```python
from build123d import *

# Parameters (mm, degrees)
SKETCH1_R               = 12.5
BOSS_EXTRUDE1_DEPTH     = 22.5
SKETCH2_R               = 7.5
CUT_EXTRUDE2_DEPTH      = 18.320508076
CUT_EXTRUDE2_DEPTH_BACK = 18.320508076
BOSS_EXTRUDE2_START     = -5
SKETCH3_R               = 12.5
BOSS_EXTRUDE2_DEPTH     = 15
SKETCH4_R               = 17.320508076
BOSS_EXTRUDE3_DEPTH     = 5


with BuildPart() as part:
    # Sketch1 → Boss-Extrude1 (new body, symmetric)
    with BuildSketch(Plane(origin=(0, 0, 0), x_dir=(0, 0, -1), z_dir=(1, 0, 0))):
        Polygon((10, 17.320508076), (-10, 17.320508076), (-20, 0), (-10, -17.320508076), (10, -17.320508076), (20, 0), align=None)
        Circle(SKETCH1_R, mode=Mode.SUBTRACT)
    extrude(amount=BOSS_EXTRUDE1_DEPTH, both=True)

    # Sketch2 → Cut-Extrude2 (cut, two sides)
    with BuildSketch(Plane(origin=(0, 0, 0), x_dir=(1, 0, 0), z_dir=(0, 1, 0))) as cut_extrude2_sk:
        Circle(SKETCH2_R)
    extrude(amount=CUT_EXTRUDE2_DEPTH, mode=Mode.SUBTRACT)
    extrude(cut_extrude2_sk.sketch, amount=-CUT_EXTRUDE2_DEPTH_BACK, mode=Mode.SUBTRACT)

    # Sketch3 → Boss-Extrude2 (add)
    with BuildSketch(Plane(origin=(22.5, 0, 0), x_dir=(0, 0, -1), z_dir=(1, 0, 0)).offset(BOSS_EXTRUDE2_START)):
        Circle(SKETCH3_R)
    boss_extrude2 = extrude(amount=BOSS_EXTRUDE2_DEPTH)

    # Sketch4 → Boss-Extrude3 (add)
    with BuildSketch(Plane(origin=(32.5, 0, 0), x_dir=(0, 0, -1), z_dir=(1, 0, 0))):
        Circle(SKETCH4_R)
    boss_extrude3 = extrude(amount=BOSS_EXTRUDE3_DEPTH)

    # Mirror3: Boss-Extrude2, Boss-Extrude3 across plane
    add(boss_extrude2.mirror(Plane(origin=(0, 0, 0), x_dir=(0, 0, 1), z_dir=(1, 0, 0))))
    add(boss_extrude3.mirror(Plane(origin=(0, 0, 0), x_dir=(0, 0, 1), z_dir=(1, 0, 0))))


solid = part.part
```
Verification items for the finished model (mm, model axes). A direction names the side the tool comes from. Coordinates: 2 decimals unless noted, no trailing zeros. Loops run counter-clockwise (first coordinate to the right, second up) from the corner with the lowest first, then second, coordinate; pieces in that order, holes last. Notation, with made-up numbers: (-28.5, -13) -> (14.5, -13) arc R13 ccw to (14.5, -5) -> close; hole circle Ø2 at (-15, -1). An arc over 180 degrees is marked (long way). Answer in a Markdown table with one row per item. Add a question column.
1. Section check C-C, the plane y = 15.5. Enter the section's corners in (x, z).
2. Draft check along X on faces 1 (the face through (37.5, 0, 0)), 2 (the face through (-7.493, -14.422, -0.33)), 3 (the face through (34.97, 5.2, -16.52)). Enter one of: +X half, -X half, draft (parallel to the pull), parting line (faces both ways), or undercut.
3. Access from +Z, -Z, +X, -X, +Y, -Y to the whole of each face (thin tool, end or side, straight path). Record for faces 4 (the face through (-34.97, 5.2, -16.52)), 5 (the face through (-0.25, 8.45, 9.21)), 6 (the face through (0.32, 8.54, -15.07)).
4. Section check A-A, the plane x = 0. Enter the section's corners in (y, z), then the cut area to 3 significant figures.
5. Material ranges on probe 1 along X at (y, z) = (14, 0); probe 2 along X at (y, z) = (1, -15.5); probe 3 along X at (y, z) = (2, 10), recorded low to high. Write a range as [from, to].
6. Section check D-D, the plane x = -13. Enter the section's corners in (y, z), then the cut area to 3 significant figures.
7. Depth check by flat-ended pin: P1, Ø3, axis at x = -19.5, y = -6.5, coming from the +Z side; P2, Ø6, axis at x = 9, z = -13.5, coming from the -Y side; P3, Ø6, axis at x = 20.5, y = -11.5, coming from the -Z side. Enter the tip coordinate at first touch or a pass-through.
Derived:
| question | item | result |
|---|---|---|
| 1 | outline | (-37.5, -7.73) -> (-32.5, -7.73) -> (-32.5, 7.73) -> (-37.5, 7.73) -> close; (-22.5, -11.05) -> (22.5, -11.05) -> (22.5, 11.05) -> (-22.5, 11.05) -> close; (32.5, -7.73) -> (37.5, -7.73) -> (37.5, 7.73) -> (32.5, 7.73) -> close; hole circle Ø15 at (0, 0) |
| 2 | face 1 | +X half |
| 2 | face 2 | undercut |
| 2 | face 3 | draft |
| 3 | face 4 | -X |
| 3 | face 5 | none |
| 3 | face 6 | -Z, +X, -X, +Y |
| 4 | outline | (-17.32, -10) -> (0, -20) -> (17.32, -10) -> (17.32, -7.5) -> (10, -7.5) arc R12.5 cw to (-10, -7.5) -> (-17.32, -7.5) -> close; (-17.32, 7.5) -> (-10, 7.5) arc R12.5 cw to (10, 7.5) -> (17.32, 7.5) -> (17.32, 10) -> (0, 20) -> (-17.32, 10) -> close |
| 4 | area | 380 mm² |
| 5 | probe 1 | x = [-37.5, -32.5], [-22.5, -7.5], [7.5, 22.5], [32.5, 37.5] |
| 5 | probe 2 | x = [-37.5, -32.5], [-22.5, 22.5], [32.5, 37.5] |
| 5 | probe 3 | x = [-37.5, -17.5], [17.5, 37.5] |
| 6 | outline | (-17.32, -10) -> (0, -20) -> (17.32, -10) -> (17.32, 10) -> (0, 20) -> (-17.32, 10) -> close; hole circle Ø25 at (0, 0) |
| 6 | area | 548 mm² |
| 7 | P1 | stops at z = 17.11 |
| 7 | P2 | stops at y = -16.45 |
| 7 | P3 | stops at z = -15.09 |
